```python
from build123d import *

# Parameters (mm, degrees)
F0_R     = 29.4132
F0_R_2   = 25.9334
F1_DEPTH = 38.1
F0_R_3   = 13.4736510141
F2_DEPTH = 59.182
F0_R_4   = 7.012968683
F3_DEPTH = 86.36
F4_DEPTH = 50.8
F0_R_5   = 3.2589999641
F5_DEPTH = 101.6


# Not quite as in the source:
# - the program builds the solid bodies; features that only make, move or delete a surface that nothing else refers to are left out


with BuildPart() as f1:
    # F0 (on Top) → F1 (new body)
    with BuildSketch(Plane.XY):
        Circle(F0_R)
        Circle(F0_R_2, mode=Mode.SUBTRACT)
    extrude(amount=F1_DEPTH)

    # F0 (on Top) → F2 (join)
    with BuildSketch(Plane.XY):
        Circle(F0_R_2)
        Circle(F0_R_3, mode=Mode.SUBTRACT)
    extrude(amount=F2_DEPTH)

    # F0 (on Top) → F3 (join)
    with BuildSketch(Plane.XY):
        Circle(F0_R_3)
        Circle(F0_R_4, mode=Mode.SUBTRACT)
    extrude(amount=F3_DEPTH)

    # F0 (on Top) → F4 (join)
    with BuildSketch(Plane.XY):
        Circle(F0_R_3)
        Circle(F0_R_4, mode=Mode.SUBTRACT)
    extrude(amount=F4_DEPTH)

    # F0 (on Top) → F5 (join)
    with BuildSketch(Plane.XY):
        Circle(F0_R_4)
        Circle(F0_R_5, mode=Mode.SUBTRACT)
    extrude(amount=F5_DEPTH)


solid = f1.part
```
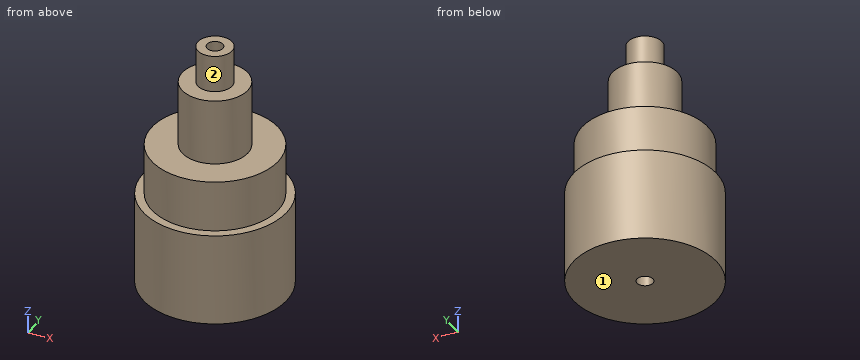
The listing builds one solid part. Answer for the finished solid, in the listing's coordinates (mm). Face numbers are marked on the shaded views. A direction names the side the tool comes from. Round coordinates to 2 decimals unless told otherwise and drop trailing zeros. Loops run counter-clockwise (first coordinate to the right, second up) from the corner with the lowest first, then second, coordinate; pieces in that order, holes last.
1) Given P1, Ø8, axis at y = -2, z = 61, coming from the +X side; P2, Ø2, axis at x = 12, y = 17, coming from the +Z side; P3, Ø1.5, axis at x = -7, z = 71, coming from the -Y side; P4, Ø10, axis at x = 6.5, y = -0.5, coming from the -Z side, each flat-ended and moving along its own axis, determine where each tip first touches the part or whether it passes through.
Outcome:
P1: stops at x = 25.93
P2: stops at z = 59.18
P3: stops at y = -11.94
P4: stops at z = 0
2) A cutting plane is placed at A-A on x = 0. Determine the outline of the cut face in (y, z).
Outcome:
outline: (-29.41, 0) - (-3.26, 0) - (-3.26, 101.6) - (-7.01, 101.6) - (-7.01, 86.36) - (-13.47, 86.36) - (-13.47, 59.18) - (-25.93, 59.18) - (-25.93, 38.1) - (-29.41, 38.1) - close; (3.26, 0) - (29.41, 0) - (29.41, 38.1) - (25.93, 38.1) - (25.93, 59.18) - (13.47, 59.18) - (13.47, 86.36) - (7.01, 86.36) - (7.01, 101.6) - (3.26, 101.6) - close
3) A cutting plane is placed at D-D on y = 24. Determine the outline of the cut face in (x, z), plus the area to 3 significant figures.
Outcome:
outline: (-17, 0) - (17, 0) - (17, 38.1) - (9.83, 38.1) - (9.83, 59.18) - (-9.83, 59.18) - (-9.83, 38.1) - (-17, 38.1) - close
area: 1,710 mm2
4) Consider line 1 (Y direction, x = 0, z = 24); line 2 (Y direction, x = 0, z = 80); line 3 (Z direction, x = 17, y = 5). Determine where each line is inside the solid, lowest interval first.
Outcome:
line 1: y = -29.41 to -3.26, 3.26 to 29.41
line 2: y = -13.47 to -3.26, 3.26 to 13.47
line 3: z = 0 to 59.18
5) A cutting plane is placed at C-C on z = 78. Determine the outline of the cut face in (x, y).
Outcome:
outline: circle Ø26.95 at (0, 0); hole circle Ø6.52 at (0, 0)
6) For the marked faces 1 and 2, determine the directions among +Z, -Z, +X, -X, +Y, -Y from which every point of the face is accessible in a straight line to the end or side of a thin tool.
Outcome:
face 1: -Z, +X, -X, +Y, -Y
face 2: +Z
